For this review, take the finished solid that the model builds, in its own axes (mm). A direction names the side the tool comes from. Round coordinates to 2 decimals unless told otherwise and drop trailing zeros. Loops run counter-clockwise (first coordinate to the right, second up) from the corner with the lowest first, then second, coordinate; pieces in that order, holes last.
```python
from build123d import *

# Parameters (mm, degrees)
SKETCH1_W                       = 22
SKETCH1_H                       = 12.7
BOSS_EXTRUDE1_DEPTH             = 26
M3X0_5_TAPPED_HOLE2_D           = 2.5
M3X0_5_TAPPED_HOLE2_DEPTH       = 5
M3X0_5_TAPPED_HOLE2_CSINK_D     = 3.05
M3X0_5_TAPPED_HOLE2_CSINK_ANGLE = 90
M3X0_5_TAPPED_HOLE2_TIP         = 0.751075774
SKETCH7_R                       = 5.7
CUT_EXTRUDE1_DEPTH              = 13.7
SKETCH8_W                       = 17
SKETCH8_H                       = 17
CUT_EXTRUDE2_DEPTH              = 4
FILLET1_R                       = 2
SKETCH9_R                       = 8.05
CUT_EXTRUDE3_DEPTH              = 2.1


with BuildPart() as part:
    # Sketch1 → Boss-Extrude1 (new body)
    with BuildSketch(Plane(origin=(0, 0, 0), x_dir=(1, 0, 0), z_dir=(0, 1, 0))):
        with Locations((11, 6.35)):
            Rectangle(SKETCH1_W, SKETCH1_H)
    extrude(amount=BOSS_EXTRUDE1_DEPTH)

    # Sketch2 → M3x0.5 Tapped Hole1 (revolve, cut)
    with BuildSketch(Plane(origin=(18, 0, -3), x_dir=(0, 0, -1), z_dir=(1, 0, 0))):
        Polygon((0, 0), (0, 5.751075774), (1.25, 5), (1.25, 0.275), (1.525, 0), align=None)
    m3x0_5_tapped_hole1 = revolve(axis=Axis((18, -6.35, -3), (0, 1, 0)), mode=Mode.SUBTRACT)

    # Mirror1: M3x0.5 Tapped Hole1 across plane
    add(m3x0_5_tapped_hole1.mirror(Plane.XY.offset(-6.35)), mode=Mode.SUBTRACT)

    # Mirror2: M3x0.5 Tapped Hole1 across plane
    add(m3x0_5_tapped_hole1.mirror(Plane(origin=(11, 0, 0), x_dir=(0, 0, 1), z_dir=(1, 0, 0))), mode=Mode.SUBTRACT)

    # Mirror2 copy 1 sketch → Mirror2 copy 1 (revolve, cut)
    with BuildSketch(Plane(origin=(4, 0, -9.7), x_dir=(0, 0, 1), z_dir=(-1, 0, 0))):
        Polygon((0, 0), (0, 5.751075774), (1.25, 5), (1.25, 0.275), (1.525, 0), align=None)
    revolve(axis=Axis((4, -6.35, -9.7), (0, 1, 0)), mode=Mode.SUBTRACT)

    # M3x0.5 Tapped Hole2
    with Locations(Plane(origin=(0, 0, 0), x_dir=(-1, 0, 0), z_dir=(0, -1, 0))):
        with Locations((-11, 6.35)):
            CounterSinkHole(M3X0_5_TAPPED_HOLE2_D / 2, M3X0_5_TAPPED_HOLE2_CSINK_D / 2, depth=M3X0_5_TAPPED_HOLE2_DEPTH, counter_sink_angle=M3X0_5_TAPPED_HOLE2_CSINK_ANGLE)
            with Locations((0, 0, -(M3X0_5_TAPPED_HOLE2_DEPTH + M3X0_5_TAPPED_HOLE2_TIP / 2))):  # 118° drill point
                Cone(0, M3X0_5_TAPPED_HOLE2_D / 2, M3X0_5_TAPPED_HOLE2_TIP, mode=Mode.SUBTRACT)

    # Sketch7 → Cut-Extrude1 (cut, through all)
    with BuildSketch(Plane.XY):
        with Locations((11, 15)):
            Circle(SKETCH7_R)
    extrude(amount=-CUT_EXTRUDE1_DEPTH, mode=Mode.SUBTRACT)

    # Sketch8 → Cut-Extrude2 (cut)
    with BuildSketch(Plane.XY):
        with Locations((11, 15)):
            Rectangle(SKETCH8_W, SKETCH8_H)
    extrude(amount=-CUT_EXTRUDE2_DEPTH, mode=Mode.SUBTRACT)

    # Fillet1
    fillet1_edges = [part.edges().sort_by_distance(p)[0] for p in [
        (2.5, 6.5, -2),
        (2.5, 23.5, -2),
        (19.5, 23.5, -2),
        (19.5, 6.5, -2),
    ]]
    fillet(fillet1_edges, radius=FILLET1_R)

    # Sketch9 → Cut-Extrude3 (cut)
    with BuildSketch(Plane(origin=(0, 0, -12.7), x_dir=(-1, 0, 0), z_dir=(0, 0, -1))):
        with Locations((-11, 15)):
            Circle(SKETCH9_R)
    extrude(amount=-CUT_EXTRUDE3_DEPTH, mode=Mode.SUBTRACT)


solid = part.part
```
(1) For faces 1 (the flat face through (2.5, 15, -2)), 2 (the cylindrical face through (12.745, 7.141, -11.665)), 3 (the cylindrical face through (14.06, 19.81, -7.25)), list the 3-axis set-ups (+Z, -Z, +X, -X, +Y, -Y) from which the entire face can be reached by the end or side of a thin tool; tool diameter is ignored.
(2) The part is to be moulded in two halves that separate along Y. For faces 4 (the flat face through (11, 23.5, -2)), 5 (the flat face through (13, 0, -6)), 6 (the flat face through (22, 13, -6)), say which applies: pulls with the +Y half, pulls with the -Y half, needs draft (parallel to the pull), parting line crosses it, or undercut.
(3) Add section A-A (y = 4.5). Give the boundary of the cut face in (x, z), plus the area to 3 significant figures.
(4) Add section D-D (y = 10). Give the boundary of the cut face in (x, z).
(5) For L1, parallel to X at y = 3.4, z = -3; L2, parallel to Z at x = 18, y = 3.7; L3, parallel to Y at x = 10.75, z = -9, list the stretches that pass through material, from the lowest coordinate up.
(6) Insertion check: pin 1 Ø3 at (x, z) = (18.5, -7.5) entering from -Y; pin 2 Ø2 at (x, z) = (4, -3) entering from -Y. Each pin has a flat end and moves straight along its axis. Give the tip position at first contact, or say it passes through.
(7) Add section B-B (z = -1). Give the boundary of the cut face in (x, y), plus the area to 3 significant figures.
(8) Add section C-C (x = 14). Give the boundary of the cut face in (y, z).
Outcome:
1. face 1: +Z
1. face 2: -Z
1. face 3: +Z, -Z
2. face 4: undercut
2. face 5: pulls with the -Y half
2. face 6: needs draft
3. outline: (0, -12.7) - (22, -12.7) - (22, 0) - (0, 0) - close; hole circle Ø2.5 at (4, -9.7); hole circle Ø2.5 at (4, -3); hole circle Ø2.5 at (11, -6.35); hole circle Ø2.5 at (18, -9.7); hole circle Ø2.5 at (18, -3)
3. area: 255 mm2
4. outline: (0, -12.7) - (4.69, -12.7) - (4.69, -10.6) - (8.26, -10.6) - (8.26, -4) - (2.5, -4) - (2.5, 0) - (0, 0) - close; (13.74, -10.6) - (17.31, -10.6) - (17.31, -12.7) - (22, -12.7) - (22, 0) - (19.5, 0) - (19.5, -4) - (13.74, -4) - close
5. L1: x = 0 to 2.75, 5.25 to 16.75, 19.25 to 22
5. L2: z = -12.7 to -10.95, -8.45 to -4.25, -1.75 to 0
5. L3: y = 0 to 9.31, 20.69 to 26
6. pin 1: stops at y = 0
6. pin 2: stops at y = 5.15
7. outline: (0, 0) - (22, 0) - (22, 26) - (0, 26) - close; hole (2.5, 8.5) arc R2 ccw to (4.5, 6.5) - (17.5, 6.5) arc R2 ccw to (19.5, 8.5) - (19.5, 21.5) arc R2 ccw to (17.5, 23.5) - (4.5, 23.5) arc R2 ccw to (2.5, 21.5) - close
7. area: 286 mm2
8. outline: (0, -12.7) - (7.53, -12.7) - (7.53, -10.6) - (10.15, -10.6) - (10.15, -4) - (6.5, -4) - (6.5, 0) - (0, 0) - close; (19.85, -10.6) - (22.47, -10.6) - (22.47, -12.7) - (26, -12.7) - (26, 0) - (23.5, 0) - (23.5, -4) - (19.85, -4) - close
